```python
from build123d import *

# Parameters (mm, degrees)
SKETCH2_R           = 3
BOSS_EXTRUDE1_DEPTH = 11
SKETCH3_R           = 4.25
BOSS_EXTRUDE2_DEPTH = 2
FILLET2_R           = 1


with BuildPart() as part:
    # Sketch2 → Boss-Extrude1 (new, symmetric)
    with BuildSketch(Plane(origin=(0, 0, 0), x_dir=(0, 0, -1), z_dir=(1, 0, 0))):
        Circle(SKETCH2_R)
    extrude(amount=BOSS_EXTRUDE1_DEPTH, both=True)

    # Sketch3 → Boss-Extrude2 (add)
    with BuildSketch(Plane(origin=(11, 0, 0), x_dir=(0, 0, -1), z_dir=(1, 0, 0))):
        Circle(SKETCH3_R)
    extrude(amount=BOSS_EXTRUDE2_DEPTH)

    # Fillet2
    fillet2_edges = [part.edges().sort_by_distance(p)[0] for p in [
        (13, 0, 4.25),
    ]]
    fillet(fillet2_edges, radius=FILLET2_R)


solid = part.part
```
Work out the finished part from the listing and answer in its coordinate system (mm). A direction names the side the tool comes from. Give positions to 0.01 mm unless a question says otherwise; leave off trailing zeros. Loops run counter-clockwise (first coordinate to the right, second up) from the corner with the lowest first, then second, coordinate; pieces in that order, holes last. Notation, with made-up numbers: (60, -40) -> (95, -40) arc R25 cw to (95, -4) -> close; hole circle Ø3 at (78.5, 81). An arc over 180 degrees is marked (long way). Put each result on its own line as item: value. Start each with the question number.
Item 1: Each of these flat-tipped pins is pushed along its axis until it touches: P1, Ø5, axis at x = 1.5, y = 1, coming from the +Z side; P2, Ø3, axis at x = 8.5, z = 0.5, coming from the +Y side; P3, Ø5, axis at x = 3, y = 2.5, coming from the -Z side. Where does it stop, or does it pass through?
Item 2: Which of the six approach directions +Z, -Z, +X, -X, +Y, -Y give full straight-line access (tool end or side, diameter ignored) to faces 1 (the face through (0, 0, 3)), 2 (the face through (11.493, 3.584, -2.285))?
Item 3: The part is cut by section C-C (x = 5.75). Give the vertices of the cut face in (y, z).
Item 4: Find the intervals of material crossed by L1, parallel to X at y = -2.5, z = 2; L2, parallel to Z at x = 9, y = -1.25; L3, parallel to Z at x = -0.25, y = -2.25, in increasing order. Write a range as [from, to].
Item 5: The part is cut by section A-A (z = 0). Give the vertices of the cut face in (x, y).
Answers below:
1. P1: z = 3
1. P2: y = 3
1. P3: z = -3
2. face 1: -X
2. face 2: +X, -X
3. outline: circle Ø6 at (0, 0)
4. L1: [11, 13]
4. L2: [-2.73, 2.73]
4. L3: [-1.98, 1.98]
5. outline: (-11, -3) -> (11, -3) -> (11, -4.25) -> (12, -4.25) arc R1 ccw to (13, -3.25) -> (13, 3.25) arc R1 ccw to (12, 4.25) -> (11, 4.25) -> (11, 3) -> (-11, 3) -> close
